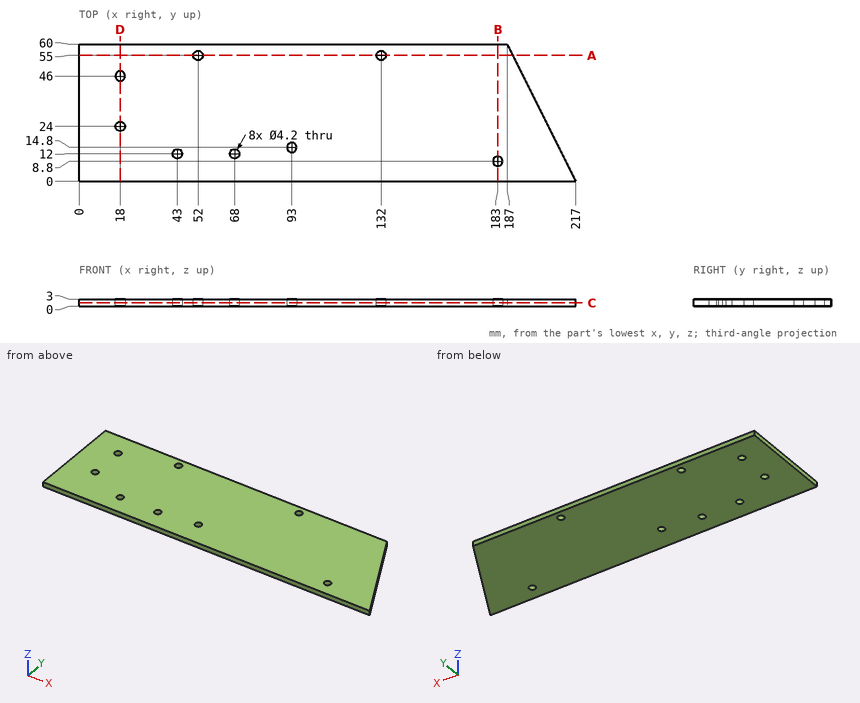
Verification items for this drawing (mm, ordinates from the low corner). Give positions to 0.01 mm unless a question says otherwise; leave off trailing zeros. Loops run counter-clockwise (first coordinate to the right, second up) from the corner with the lowest first, then second, coordinate; pieces in that order, holes last.
1. Material ranges on probe 1 along Y at (x, z) = (18, 0.9); probe 2 along Y at (x, z) = (183, 1.55); probe 3 along X at (y, z) = (13.5, 2.45), recorded low to high.
Derived:
probe 1: y = 0 to 21.9, 26.1 to 43.9, 48.1 to 60
probe 2: y = 0 to 6.7, 10.9 to 60
probe 3: x = 0 to 41.53, 44.47 to 66.53, 69.47 to 91.35, 94.65 to 210.25
2. Cross-section at D-D on x = 18. Record the cut outline in (y, z), and give its area (3 significant figures).
Derived:
outline: (0, 0) - (21.9, 0) - (21.9, 3) - (0, 3) - close; (26.1, 0) - (43.9, 0) - (43.9, 3) - (26.1, 3) - close; (48.1, 0) - (60, 0) - (60, 3) - (48.1, 3) - close
area: 155 mm2
3. Cross-section at B-B on x = 183. Record the cut outline in (y, z), and give its area (3 significant figures).
Derived:
outline: (0, 0) - (6.7, 0) - (6.7, 3) - (0, 3) - close; (10.9, 0) - (60, 0) - (60, 3) - (10.9, 3) - close
area: 167 mm2
4. Cross-section at A-A on y = 55. Record the cut outline in (x, z), and give its area (3 significant figures).
Derived:
outline: (0, 0) - (49.9, 0) - (49.9, 3) - (0, 3) - close; (54.1, 0) - (129.9, 0) - (129.9, 3) - (54.1, 3) - close; (134.1, 0) - (189.5, 0) - (189.5, 3) - (134.1, 3) - close
area: 543 mm2
5. Go/stop test with flat-tipped pins: P1, Ø5.5, axis at x = 132, y = 55, coming from the +Z side; P2, Ø3.5, axis at x = 183, y = 8.8, coming from the +Z side. Record where each tip stops, or that it passes through.
Derived:
P1: stops at z = 3
P2: passes through
6. Cross-section at C-C on z = 1.5. Count the separate pieces of the cut face and the enclosed holes in it, and give its area (3 significant figures).
Derived:
separate pieces: 1
enclosed holes: 8
area: 12,000 mm2
